Autodesk Inventor part; units mm, degrees
ref_plane "YZ Plane" through (0, 0, 0) normal (1, 0, 0) x (0, 1, 0)
ref_plane "XZ Plane" through (0, 0, 0) normal (0, 1, 0) x (-1, 0, 0)
ref_plane "XY Plane" through (0, 0, 0) normal (0, 0, 1) x (1, 0, 0)
sketch "Esboço1" plane through (0, 0, 0) normal (1, 0, 0) x (0, 1, 0)
  line L0 (0, 0) -> (29, 0)
  line L1 (29, 0) -> (29, -15)
  line L2 (29, -15) -> (14, -15)
  line L3 (14, -15) -> (0, -12.5)
  line L4 (0, -12.5) -> (0, -9)
  line L5 (0, -9) -> (9.7213, -9)
  arc A0 (9, -9) -> (18, 0) centre (9, 0) ccw
  point P0 (4.8606, -9)
  dimension "d0" = 15
  dimension "d1" = 12.5
  dimension "d2" = 15
  dimension "d3" = 29
  dimension "d5" = 9
  dimension "d7" = 9
revolve "Revolução1" add sketch "Esboço1" angle 360 about axis through (0, 0, 0) along (0, 1, 0)
sketch "Esboço2" plane through (0, 0, 0) normal (0, 0, 1) x (1, 0, 0)
  line L0 (0, 0) -> (0, 39.2335)
  line L1 (-2.5, 3) -> (2.5, 3)
  line L2 (2.5, 3) -> (2.5, -0.6056)
  line L3 (2.5, -0.6056) -> (-2.5, -0.6056)
  line L4 (-2.5, -0.6056) -> (-2.5, 3)
  line L5 (12.5, 0) -> (-12.5, 0)
  dimension "d9" = 5
  dimension "d10" = 2.5
  dimension "d11" = 3
extrude "Extrusão1" cut sketch "Esboço2" along normal through all both and the other way through all
pattern_circular "Padrão circular1" count 4 over 360 about axis through (0, 21.5, 0) along (0, 1, 0) of "Extrusão1"
sketch "Esboço3" plane through (0, 0, 0) normal (0, 0, 1) x (1, 0, 0)
  line L0 (15, 29) -> (-15, 29)
  line L1 (-7, 29) -> (0, 22)
  line L2 (0, 22) -> (7, 29)
  line L3 (-7, 29) -> (7, 29)
  line L4 (0, 29) -> (0, 9.5937)
  line L5 (2.5, 0) -> (2.5, 3)
  point P0 (0, 0)
  dimension "d17" = 45
  dimension "d19" = 2.5
  dimension "d20" = 7
extrude "Extrusão2" cut sketch "Esboço3" along normal through all both and the other way through all
sketch "Esboço4" plane through (0, 0, 0) normal (1, 0, 0) x (0, 1, 0)
  line L0 (29, -13.2665) -> (29, 13.2665)
  line L1 (29, -2) -> (27, 0)
  line L2 (27, 0) -> (29, 2)
  line L3 (29, -2) -> (29, 2)
  line L4 (3, -2.5) -> (3, 2.5)
  line L5 (3, 0) -> (30.8136, 0)
  point P0 (0, 0)
  dimension "d23" = 2
  dimension "d24" = 45
  dimension "d25" = 45
extrude "Extrusão3" cut sketch "Esboço4" along normal through all both and the other way through all
pattern_linear "Padrão retangular1" count 4 spacing 4 along (0, 0, 1) of "Extrusão3"
pattern_linear "Padrão retangular2" count 4 spacing 4 along (0, 0, -1) of "Extrusão3"
properties part number "CHAPEU" material "Latão, amarelo macio"
Could you check a few things on this model? Use its own coordinates, in mm. A direction names the side the tool comes from. Coordinates: 2 decimals unless noted, no trailing zeros. Loops run counter-clockwise (first coordinate to the right, second up) from the corner with the lowest first, then second, coordinate; pieces in that order, holes last.
1) Imagine slicing it at A-A (y = 7). List the corners of the cut face in (x, z) for me.
Reported:
outline: circle Ø27.5 at (0, 0); hole circle Ø18 at (0, 0)
2) Will these pins go through, and if not, where does the flat tip stop? pin 1 Ø3.5 at (y, z) = (1.5, -11.5) entering from +X; pin 2 Ø0.9 at (y, z) = (1.5, 11) entering from -X; pin 3 Ø1.5 at (x, z) = (-11, -0.5) entering from +Y.
Reported:
pin 1: stops at x = 8.3
pin 2: stops at x = -7.21
pin 3: stops at y = 28.25
3) Which directions (+Z, -Z, +X, -X, +Y, -Y) give clear straight access to the entire face, cutting with the end or side of a thin tool? Please do faces 4 (the face through (11, 1, 2.5)), 5 (the face through (-9, 28, -7)), 6 (the face through (0, 3, 11)).
Reported:
face 4: +X, -X, -Y
face 5: +X, -X, +Y
face 6: +Z, -Z, -Y
4) Thinking about a two-plate mould opening in Z: for faces 1 (the face through (-3, 25, 0)), 2 (the face through (11.97, 5.54, -6.22)), 3 (the face through (-10, 28, 3)), which applies, released by +Z, released by -Z, zero draft, split by the parting line, or undercut?
Reported:
face 1: zero draft
face 2: split by the parting line
face 3: undercut
5) Please list where these lines run through material, in increasing order: line 1 along Z through (x, y) = (0.25, 11); line 2 along X through (y, z) = (5.5, 0); line 3 along X through (y, z) = (7.5, -3.75).
Reported:
line 1: z = -14.46 to -8.77, 8.77 to 14.46
line 2: x = -13.48 to -9, 9 to 13.48
line 3: x = -13.32 to -8.18, 8.18 to 13.32
6) Imagine slicing it at B-B (y = 20.5). List the corners of the cut face in (x, z) for me, and give its area (3 significant figures).
Reported:
outline: circle Ø30 at (0, 0)
area: 707 mm2
7) Imagine slicing it at C-C (y = 26.5). List the corners of the cut face in (x, z) for me.
Reported:
outline: (-4.5, -14.31) - (-4.5, 14.31) arc R15 ccw to start; (4.5, -14.31) arc R15 ccw to (4.5, 14.31) - close
